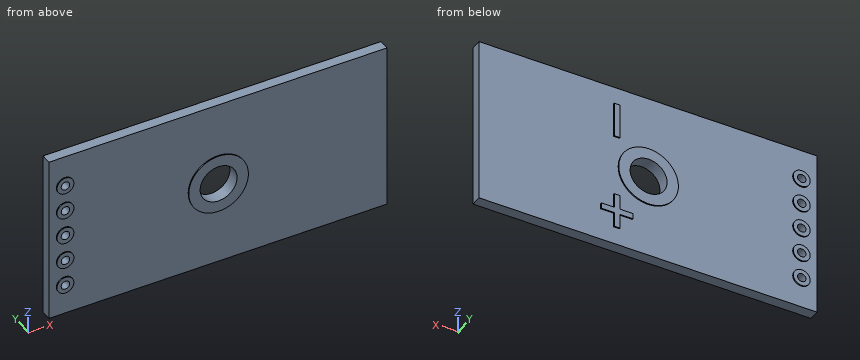
```python
from build123d import *

# Parameters (mm, degrees)
SKETCH1_W                = 32
SKETCH1_H                = 16
BOSS_EXTRUDE1_DEPTH      = 1
SKETCH2_R                = 1.75
SKETCH2_R_2              = 0.4
CUT_EXTRUDE1_DEPTH       = 1
BOSS_EXTRUDE2_DEPTH      = 0.1
BOSS_EXTRUDE2_DEPTH_BACK = 1.1
SKETCH3_R                = 0.8
SKETCH3_R_2              = 0.4
SKETCH3_R_3              = 2.823446158
SKETCH3_R_4              = 1.75
SKETCH4_W                = 0.541769891
SKETCH4_H                = 3.328015046
BOSS_EXTRUDE3_DEPTH      = 0.1


with BuildPart() as part:
    # Sketch1 → Boss-Extrude1 (new body)
    with BuildSketch(Plane(origin=(0, 0, 0), x_dir=(1, 0, 0), z_dir=(0, 1, 0))):
        Rectangle(SKETCH1_W, SKETCH1_H)
    extrude(amount=BOSS_EXTRUDE1_DEPTH)

    # Sketch2 → Cut-Extrude1 (cut)
    with BuildSketch(Plane(origin=(0, 1, 0), x_dir=(1, 0, 0), z_dir=(0, 1, 0))):
        with Locations(Location((0, 0, 0), (0, 0, 270))):
            Circle(SKETCH2_R)
        with Locations(Location((-14.5, -5.08, 0), (0, 0, 270))):
            Circle(SKETCH2_R_2)
        with Locations(Location((-14.5, -2.54, 0), (0, 0, 270))):
            Circle(SKETCH2_R_2)
        with Locations(Location((-14.5, 0, 0), (0, 0, 270))):
            Circle(SKETCH2_R_2)
        with Locations(Location((-14.5, 2.54, 0), (0, 0, 270))):
            Circle(SKETCH2_R_2)
        with Locations(Location((-14.5, 5.08, 0), (0, 0, 270))):
            Circle(SKETCH2_R_2)
    extrude(amount=-CUT_EXTRUDE1_DEPTH, mode=Mode.SUBTRACT)

    # Sketch3 → Boss-Extrude2 (add, two sides: drawn at the far end of the back side and taken through both)
    # profile 1 of 6: a face of its own
    with BuildSketch(Plane(origin=(0, 1, 0), x_dir=(1, 0, 0), z_dir=(0, 1, 0)).offset(-BOSS_EXTRUDE2_DEPTH_BACK)):
        with Locations(Location((-14.5, 5.08, 0), (0, 0, 270))):
            Circle(SKETCH3_R)
        with Locations(Location((-14.5, 5.08, 0), (0, 0, 270))):
            Circle(SKETCH3_R_2, mode=Mode.SUBTRACT)
    # profile 2 of 6: a face of its own
    with BuildSketch(Plane(origin=(0, 1, 0), x_dir=(1, 0, 0), z_dir=(0, 1, 0)).offset(-BOSS_EXTRUDE2_DEPTH_BACK)):
        with Locations(Location((-14.5, 2.54, 0), (0, 0, 270))):
            Circle(SKETCH3_R)
        with Locations(Location((-14.5, 2.54, 0), (0, 0, 270))):
            Circle(SKETCH3_R_2, mode=Mode.SUBTRACT)
    # profile 3 of 6: a face of its own
    with BuildSketch(Plane(origin=(0, 1, 0), x_dir=(1, 0, 0), z_dir=(0, 1, 0)).offset(-BOSS_EXTRUDE2_DEPTH_BACK)):
        with Locations(Location((-14.5, 0, 0), (0, 0, 270))):
            Circle(SKETCH3_R)
        with Locations(Location((-14.5, 0, 0), (0, 0, 270))):
            Circle(SKETCH3_R_2, mode=Mode.SUBTRACT)
    # profile 4 of 6: a face of its own
    with BuildSketch(Plane(origin=(0, 1, 0), x_dir=(1, 0, 0), z_dir=(0, 1, 0)).offset(-BOSS_EXTRUDE2_DEPTH_BACK)):
        with Locations(Location((-14.5, -2.54, 0), (0, 0, 270))):
            Circle(SKETCH3_R)
        with Locations(Location((-14.5, -2.54, 0), (0, 0, 270))):
            Circle(SKETCH3_R_2, mode=Mode.SUBTRACT)
    # profile 5 of 6: a face of its own
    with BuildSketch(Plane(origin=(0, 1, 0), x_dir=(1, 0, 0), z_dir=(0, 1, 0)).offset(-BOSS_EXTRUDE2_DEPTH_BACK)):
        with Locations(Location((-14.5, -5.08, 0), (0, 0, 270))):
            Circle(SKETCH3_R)
        with Locations(Location((-14.5, -5.08, 0), (0, 0, 270))):
            Circle(SKETCH3_R_2, mode=Mode.SUBTRACT)
    # profile 6 of 6: a face of its own
    with BuildSketch(Plane(origin=(0, 1, 0), x_dir=(1, 0, 0), z_dir=(0, 1, 0)).offset(-BOSS_EXTRUDE2_DEPTH_BACK)):
        with Locations(Location((0, 0, 0), (0, 0, 270))):
            Circle(SKETCH3_R_3)
        with Locations(Location((0, 0, 0), (0, 0, 270))):
            Circle(SKETCH3_R_4, mode=Mode.SUBTRACT)
    extrude(amount=BOSS_EXTRUDE2_DEPTH + BOSS_EXTRUDE2_DEPTH_BACK)

    # Sketch4 → Boss-Extrude3 (add)
    with BuildSketch(Plane(origin=(0, 1, 0), x_dir=(1, 0, 0), z_dir=(0, 1, 0))):
        Polygon((3.250619348, 6.3), (3.250619348, 4.905884946), (4.479734402, 4.905884946), (4.479734402, 4.364115054), (3.250619348, 4.364115054), (3.250619348, 2.97), (2.708849457, 2.97), (2.708849457, 4.364115054), (1.479734402, 4.364115054), (1.479734402, 4.905884946), (2.708849457, 4.905884946), (2.708849457, 6.3), align=None)
        with Locations((2.979734403, -4.634884299)):
            Rectangle(SKETCH4_W, SKETCH4_H)
    extrude(amount=BOSS_EXTRUDE3_DEPTH)


solid = part.part
```
Part model, mm, in its own coordinate system. Round coordinates to 2 decimals unless told otherwise and drop trailing zeros. Loops run counter-clockwise (first coordinate to the right, second up) from the corner with the lowest first, then second, coordinate; pieces in that order, holes last. Notation, with made-up numbers: (-17.5, -30) -> (25.5, -30) arc R10 cw to (25.5, -17) -> close; hole circle Ø2 at (88, -15.75). An arc over 180 degrees is marked (long way). Use a Markdown table: item, result.
1) Cut at C-C, the plane x = -1. List the corners of the cut face in (y, z).
The answers:
| item | result |
|---|---|
| outline | (-0.1, -2.64) -> (0, -2.64) -> (0, -8) -> (1, -8) -> (1, -2.64) -> (1.1, -2.64) -> (1.1, -1.44) -> (-0.1, -1.44) -> close; (-0.1, 1.44) -> (1.1, 1.44) -> (1.1, 2.64) -> (1, 2.64) -> (1, 8) -> (0, 8) -> (0, 2.64) -> (-0.1, 2.64) -> close |
2) Cut at A-A, the plane z = 5.08. List the corners of the cut face in (x, y), and give its area (3 significant figures).
The answers:
| item | result |
|---|---|
| outline | (-16, 0) -> (-15.3, 0) -> (-15.3, -0.1) -> (-14.9, -0.1) -> (-14.9, 1.1) -> (-15.3, 1.1) -> (-15.3, 1) -> (-16, 1) -> close; (-14.1, -0.1) -> (-13.7, -0.1) -> (-13.7, 0) -> (16, 0) -> (16, 1) -> (3.25, 1) -> (3.25, 1.1) -> (2.71, 1.1) -> (2.71, 1) -> (-13.7, 1) -> (-13.7, 1.1) -> (-14.1, 1.1) -> close |
| area | 31.4 mm2 |
3) Cut at D-D, the plane z = 0. List the corners of the cut face in (x, y), and give its area (3 significant figures).
The answers:
| item | result |
|---|---|
| outline | (-16, 0) -> (-15.3, 0) -> (-15.3, -0.1) -> (-14.9, -0.1) -> (-14.9, 1.1) -> (-15.3, 1.1) -> (-15.3, 1) -> (-16, 1) -> close; (-14.1, -0.1) -> (-13.7, -0.1) -> (-13.7, 0) -> (-2.82, 0) -> (-2.82, -0.1) -> (-1.75, -0.1) -> (-1.75, 1.1) -> (-2.82, 1.1) -> (-2.82, 1) -> (-13.7, 1) -> (-13.7, 1.1) -> (-14.1, 1.1) -> close; (1.75, -0.1) -> (2.82, -0.1) -> (2.82, 0) -> (16, 0) -> (16, 1) -> (2.82, 1) -> (2.82, 1.1) -> (1.75, 1.1) -> close |
| area | 28.3 mm2 |
4) Probe line 1 (X direction, y = 0.7, z = 0); line 2 (X direction, y = 0.45, z = 2.54); line 3 (Y direction, x = -8.5, z = 4.5). List the from-to ranges inside material, lowest first. Write a range as [from, to].
The answers:
| item | result |
|---|---|
| line 1 | x = [-16, -14.9], [-14.1, -1.75], [1.75, 16] |
| line 2 | x = [-16, -14.9], [-14.1, 16] |
| line 3 | y = [0, 1] |
5) Drop flat-ended pins along their axis: pin 1 Ø2 at (x, z) = (0, 0) entering from -Y; pin 2 Ø5 at (x, z) = (6, 0.5) entering from -Y; pin 3 Ø8 at (x, z) = (0, -4) entering from -Y; pin 4 Ø1.5 at (x, z) = (-7, 6.5) entering from +Y. Give the stop position or say it passes through.
The answers:
| item | result |
|---|---|
| pin 1 | passes through |
| pin 2 | stops at y = 0 |
| pin 3 | stops at y = -0.1 |
| pin 4 | stops at y = 1 |
6) Cut at B-B, the plane y = 0.4. List the corners of the cut face in (x, z).
The answers:
| item | result |
|---|---|
| outline | (-16, -8) -> (16, -8) -> (16, 8) -> (-16, 8) -> close; hole circle Ø0.8 at (-14.5, -5.08); hole circle Ø0.8 at (-14.5, -2.54); hole circle Ø0.8 at (-14.5, 0); hole circle Ø0.8 at (-14.5, 2.54); hole circle Ø0.8 at (-14.5, 5.08); hole circle Ø3.5 at (0, 0) |
